Read the model definition and answer for the solid it produces. Units are mm, in the model's axes. A direction names the side the tool comes from. Give positions to 0.01 mm unless a question says otherwise; leave off trailing zeros. Order: outer loops, then holes, each group sorted by start corner. A loop starts at its lowest first (then second) coordinate and runs counter-clockwise, first axis right, second up. Notation, with made-up numbers: M -37,43 L 21,43 A12 ccw 21,58 Z; hole C 79,18 d1. An arc over 180 degrees is marked long. One line per item, written item: value. Start each with the question number.
from build123d import *

# Parameters (mm, degrees)
SKETCH1_W           = 60
SKETCH1_H           = 30
BOSS_EXTRUDE1_DEPTH = 8
SKETCH3_W           = 10
SKETCH3_H           = 30
BOSS_EXTRUDE5_DEPTH = 7
SKETCH5_W           = 14
SKETCH5_H           = 30
BOSS_EXTRUDE6_DEPTH = 11
SKETCH6_R           = 5
CUT_EXTRUDE1_DEPTH  = 69.738635424
FILLET1_R           = 7
FILLET2_R           = 5
FILLET3_R           = 5
BOSS_EXTRUDE7_DEPTH = 30


with BuildPart() as part:
    # Sketch1 → Boss-Extrude1 (new body)
    with BuildSketch(Plane(origin=(0, 0, 0), x_dir=(1, 0, 0), z_dir=(0, 1, 0))):
        with Locations((30, 15)):
            Rectangle(SKETCH1_W, SKETCH1_H)
    extrude(amount=BOSS_EXTRUDE1_DEPTH)

    # Sketch3 → Boss-Extrude5 (add)
    with BuildSketch(Plane(origin=(0, 8, 0), x_dir=(1, 0, 0), z_dir=(0, 1, 0))):
        with Locations((30, 15)):
            Rectangle(SKETCH3_W, SKETCH3_H)
    extrude(amount=BOSS_EXTRUDE5_DEPTH)

    # Sketch5 → Boss-Extrude6 (add)
    with BuildSketch(Plane.XZ):
        with Locations((30, -15)):
            Rectangle(SKETCH5_W, SKETCH5_H)
    extrude(amount=BOSS_EXTRUDE6_DEPTH)

    # Sketch6 → Cut-Extrude1 (cut, through all)
    with BuildSketch(Plane(origin=(0, 0, -30), x_dir=(-1, 0, 0), z_dir=(0, 0, -1))):
        with Locations((-30, -5)):
            Circle(SKETCH6_R)
    extrude(amount=-CUT_EXTRUDE1_DEPTH, mode=Mode.SUBTRACT)

    # Fillet1
    fillet1_edges = [part.edges().sort_by_distance(p)[0] for p in [
        (23, -11, -15),
        (37, -11, -15),
    ]]
    fillet(fillet1_edges, radius=FILLET1_R - 0.0001)  # a hair under: the kernel refuses the full size

    # Fillet2
    fillet2_edges = [part.edges().sort_by_distance(p)[0] for p in [
        (23, 0, -15),
    ]]
    fillet(fillet2_edges, radius=FILLET2_R)

    # Fillet3
    fillet3_edges = [part.edges().sort_by_distance(p)[0] for p in [
        (37, 0, -15),
    ]]
    fillet(fillet3_edges, radius=FILLET3_R)

    # Sketch8 → Boss-Extrude7 (add)
    with BuildSketch(Plane(origin=(0, 0, -30), x_dir=(-1, 0, 0), z_dir=(0, 0, -1))):
        with BuildLine():
            Line((-41.958260743, -1), (-42.958260743, 0))
            Line((-42.958260743, 0), (-41.958260743, 0))
            ThreePointArc((-41.958260743, 0), (-38.573244741, -1.320099639), (-36.9756521, -4.583333333))
            ThreePointArc((-36.9756521, -4.583333333), (-34.739022403, -9.151860505), (-30, -11))
            ThreePointArc((-30, -11), (-25.260977597, -9.151860505), (-23.0243479, -4.583333333))
            ThreePointArc((-23.0243479, -4.583333333), (-21.426755259, -1.320099639), (-18.041739257, 0))
            Line((-18.041739257, 0), (-16.803044796, 0))
            Line((-16.803044796, 0), (-18.041739257, -1))
            ThreePointArc((-18.041739257, -1), (-20.749752058, -2.056079711), (-22.027826171, -4.666666667))
            ThreePointArc((-22.027826171, -4.666666667), (-24.583974397, -9.887840578), (-30, -12))
            ThreePointArc((-30, -12), (-35.416025603, -9.887840578), (-37.972173829, -4.666666667))
            ThreePointArc((-37.972173829, -4.666666667), (-39.250247942, -2.056079711), (-41.958260743, -1))
        make_face()
    extrude(amount=-BOSS_EXTRUDE7_DEPTH)


solid = part.part
Q1. Determine the mould class of faces 1 (the cylindrical face through (20.72, -2.03, -15.21)), 2 (the flat face through (30, 5, -30)), 3 (the cylindrical face through (35, -5, -15)), 4 (the flat face through (47, 8, -15)) for opening direction Y: released by +Y, released by -Y, zero draft, split by the parting line, or undercut.
Q2. Find section A-A, the plane x = 29. Give the vertices of the cut face in (y, z).
Q3. A tool of negligible diameter and unlimited length cuts with its end or side. For faces 5 (the flat face through (35, 11, -15)), 6 (the flat face through (8, 0, -15)), 7 (the flat face through (25, 11, -15)), from which of +Z, -Z, +X, -X, +Y, -Y can it reach the whole face along a straight path? Write none if from no direction.
Q4. Find section B-B, the plane z = -8. Give the vertices of the cut face in (x, y).
Q5. Find section C-C, the plane y = -2. Give the vertices of the cut face in (x, z), then the cut area to 3 significant figures.
Q6. Consider probe 1 along Y at (x, z) = (30, -19.5); probe 2 along Y at (x, z) = (9, -19.5); probe 3 along X at (y, z) = (-0.5, -24.25). Determine where each line is inside the solid, lowest interval first.
Q7. Find section D-D, the plane x = 45. Give the vertices of the cut face in (y, z), then the cut area to 3 significant figures.
Q8. Each of these flat-tipped pins is pushed along its axis until it touches: pin 1 (8 mm diameter, centred on x = 29.5, z = -18.5, fed in from -Y); pin 2 (6 mm diameter, centred on x = 43, z = -8.5, fed in from +Y); pin 3 (4 mm diameter, centred on x = 41, z = -4.5, fed in from -Y); pin 4 (8 mm diameter, centred on x = 39.5, z = -23.5, fed in from -Y). Where does it stop, or does it pass through?
Evaluation:
1. face 1: released by -Y
1. face 2: zero draft
1. face 3: undercut
1. face 4: released by +Y
2. outline: M -11.94,-30 L -9.9,-30 L -9.9,0 L -11.94,0 Z; M -0.1,-30 L 15,-30 L 15,0 L -0.1,0 Z
3. face 5: +Z, -Z, +X, +Y
3. face 6: +Z, -Z, -X, -Y
3. face 7: +Z, -Z, -X, +Y
4. outline: M 0,0 L 16.8,0 L 18.04,-1 A4 cw 22.03,-4.67 A8 ccw 37.97,-4.67 A4 cw 41.96,-1 L 42.96,0 L 60,0 L 60,8 L 35,8 L 35,15 L 25,15 L 25,8 L 0,8 Z; hole C 30,-5 d10
5. outline: M 20.69,-30 L 26,-30 L 26,0 L 20.69,0 Z; M 34,-30 L 39.31,-30 L 39.31,0 L 34,0 Z
5. area: 319 mm2
6. probe 1: -12 to -10, 0 to 15
6. probe 2: 0 to 8
6. probe 3: 17.42 to 27.82, 32.18 to 42.46
7. outline: M 0,-30 L 8,-30 L 8,0 L 0,0 Z
7. area: 240 mm2
8. pin 1: y = -12
8. pin 2: y = 8
8. pin 3: y = -2.31
8. pin 4: y = -9.81
